```python
from build123d import *

# Parameters (mm, degrees)
SKETCH2_R          = 11.5
EXTRUDE1_DEPTH     = 20
SKETCH3_R          = 9
EXTRUDE2_DEPTH     = 14
SKETCH4_R          = 7.5
EXTRUDE3_DEPTH     = 20
SKETCH5_R          = 6
EXTRUDE4_DEPTH     = 15
EXTRUDE5_START     = 100
SKETCH6_R          = 9
EXTRUDE5_DEPTH     = 100
EXTRUDE6_START     = 12
SKETCH7_R          = 6
EXTRUDE6_DEPTH     = 12
SCALE1_SCALE       = 5
SKETCH9_W          = 32
SKETCH9_H          = 18
CUT_EXTRUDE1_DEPTH = 665.990601438
CUT_EXTRUDE2_DEPTH = 481.888860648
CUT_EXTRUDE3_DEPTH = 483.218372884
CHAMFER1_SIZE      = 2
SKETCH12_W         = 80
SKETCH12_H         = 80
SKETCH12_W_2       = 45
SKETCH12_H_2       = 45
CUT_EXTRUDE4_DEPTH = 50


with BuildPart() as part:
    # Sketch2 → Extrude1 (new body)
    with BuildSketch(Plane(origin=(0, 0, 0), x_dir=(0, 0, -1), z_dir=(1, 0, 0))):
        Circle(SKETCH2_R)
    extrude(amount=EXTRUDE1_DEPTH)

    # Sketch3 → Extrude2 (add)
    with BuildSketch(Plane(origin=(20, 0, 0), x_dir=(0, 0, -1), z_dir=(1, 0, 0))):
        Circle(SKETCH3_R)
    extrude(amount=EXTRUDE2_DEPTH)

    # Sketch4 → Extrude3 (add)
    with BuildSketch(Plane(origin=(34, 0, 0), x_dir=(0, 0, -1), z_dir=(1, 0, 0))):
        Circle(SKETCH4_R)
    extrude(amount=EXTRUDE3_DEPTH)

    # Sketch5 → Extrude4 (add)
    with BuildSketch(Plane(origin=(54, 0, 0), x_dir=(0, 0, -1), z_dir=(1, 0, 0))):
        Circle(SKETCH5_R)
    extrude(amount=EXTRUDE4_DEPTH)

    # Sketch6 → Extrude5 (add)
    with BuildSketch(Plane.ZY.offset(EXTRUDE5_START)):
        with Locations(Location((0, 0, 0), (0, 0, 180))):
            Circle(SKETCH6_R)
    extrude(amount=-EXTRUDE5_DEPTH)

    # Sketch7 → Extrude6 (add)
    with BuildSketch(Plane.ZY.offset(100).offset(EXTRUDE6_START)):
        with Locations(Location((0, 0, 0), (0, 0, 180))):
            Circle(SKETCH7_R)
    extrude(amount=-EXTRUDE6_DEPTH)


with BuildPart() as part_1:
    # Scale1: scaled about (-22.253434459, 0, 0)
    add(part.part.scale(SCALE1_SCALE).moved(Location((89.013737836, 0, 0))))

    # Sketch9 → Cut-Extrude1 (cut, through all)
    with BuildSketch(Plane(origin=(189.013737836, 0, 0), x_dir=(0, 0, -1), z_dir=(1, 0, 0))):
        with Locations((0, 55.5)):
            Rectangle(SKETCH9_W, SKETCH9_H)
    cut_extrude1 = extrude(amount=-CUT_EXTRUDE1_DEPTH, mode=Mode.SUBTRACT)

    # Mirror1: Cut-Extrude1 across plane
    add(cut_extrude1.mirror(Plane.ZX), mode=Mode.SUBTRACT)

    # Sketch10 → Cut-Extrude2 (cut, through all)
    with BuildSketch(Plane(origin=(0, 23, 0), x_dir=(-1, 0, 0), z_dir=(0, 1, 0))):
        with BuildLine():
            Line((-373.013737836, -9), (-434.013737836, -9))
            Line((-434.013737836, -9), (-434.013737836, 9))
            Line((-434.013737836, 9), (-373.013737836, 9))
            ThreePointArc((-373.013737836, 9), (-364.013737836, 0), (-373.013737836, -9))
        make_face()
    extrude(amount=CUT_EXTRUDE2_DEPTH, mode=Mode.SUBTRACT)

    # Sketch11 → Cut-Extrude3 (cut, through all)
    with BuildSketch(Plane(origin=(0, 0, 30), x_dir=(-1, 0, 0), z_dir=(0, 0, 1))):
        with BuildLine():
            Line((-339.013737836, 10), (-279.013737836, 10))
            ThreePointArc((-279.013737836, 10), (-269.013737836, 0), (-279.013737836, -10))
            Line((-279.013737836, -10), (-339.013737836, -10))
            ThreePointArc((-339.013737836, -10), (-349.013737836, 0), (-339.013737836, 10))
        make_face()
    extrude(amount=CUT_EXTRUDE3_DEPTH, mode=Mode.SUBTRACT)

    # Chamfer1
    chamfer1_edges = [part_1.edges().sort_by_distance(p)[0] for p in [
        (-470.986262164, 0, 30),
    ]]
    chamfer(chamfer1_edges, length=CHAMFER1_SIZE)

    # Sketch12 → Cut-Extrude4 (cut)
    with BuildSketch(Plane.ZY.offset(470.986262164)):
        Rectangle(SKETCH12_W, SKETCH12_H)
        Rectangle(SKETCH12_W_2, SKETCH12_H_2, mode=Mode.SUBTRACT)
    extrude(amount=-CUT_EXTRUDE4_DEPTH, mode=Mode.SUBTRACT)


solid = part_1.part
```
Here's how the part is built. I have some questions about the finished solid (model axes, mm). A direction names the side the tool comes from. Coordinates: 2 decimals unless noted, no trailing zeros. Loops run counter-clockwise (first coordinate to the right, second up) from the corner with the lowest first, then second, coordinate; pieces in that order, holes last. Notation, with made-up numbers: (20, 7) - (34, 7) arc R26 ccw to (34, 46) - close; hole circle Ø11 at (-39, 6). An arc over 180 degrees is marked (long way). Return JSON: item names as keys, results as strings. Group by question number.
Item 1: Will these pins go through, and if not, where does the flat tip stop? P1, Ø1, axis at x = -224, z = -9.5, coming from the -Y side; P2, Ø4.5, axis at x = 402, y = 26, coming from the -Z side; P3, Ø2.5, axis at x = 115.5, y = 51.5, coming from the +Z side.
Item 2: On a 3-axis mill with a long thin cutter (end or side, diameter ignored), from which of +Z, -Z, +X, -X, +Y, -Y can I reach the whole of each face in a straight line? I mean faces 4 (the face through (223.524, -39.923, -20.765)), 5 (the face through (-446, 0, -22.5)), 6 (the face through (-410.986, 29, -9)). Say none if no direction works.
Item 3: We'd pull the mould along X, two halves only. Please class faces 1 (the face through (308, 0, 30)), 2 (the face through (-446, 0, 22.5)), 3 (the face through (189.014, -45, -8)): +X half, -X half, draft (parallel to the pull), parting line (faces both ways), or undercut.
Item 4: If we section it at C-C on x = -127: Write out the boundary of the cut face in (y, z).
Item 5: I need wall thicknesses on line 1 (X direction, y = -17.5, z = 49); line 2 (Y direction, x = -204.5, z = 1); line 3 (X direction, y = -34.5, z = -21.5). Which ranges of each line are inside material? Lowest first, please. Write a range as from..to.
Calculated:
{
 "1": {"P1": "stops at y = -44.09", "P2": "stops at z = -18.33", "P3": "stops at z = 27.95"},
 "2": {"face 4": "+X", "face 5": "-Z, -X, +Y, -Y", "face 6": "-X"},
 "3": {"face 1": "undercut", "face 2": "draft", "face 3": "+X half"},
 "4": {"outline": "circle Ø90 at (0, 0)"},
 "5": {"line 1": "x = 89.01..189.01", "line 2": "y = -44.99..44.99", "line 3": "x = -410.99..259.01"}
}
